```python
from build123d import *

# Parameters (mm, degrees)
F0_W     = 1300
F0_H     = 500
F0_W_2   = 1140
F0_H_2   = 340
F1_DEPTH = 200
F3_DEPTH = 345
F5_DEPTH = 40
F7_DEPTH = 35


# Not quite as in the source:
# - a feature names something its author has since deleted; it is built from what else it names


with BuildPart() as f1:
    # F0 (on Top) → F1 (new body)
    with BuildSketch(Plane.XY):
        Rectangle(F0_W, F0_H)
        Rectangle(F0_W_2, F0_H_2, mode=Mode.SUBTRACT)
    extrude(amount=F1_DEPTH)



with BuildPart() as f3:
    # F2 (on Front) → F3 (new body, symmetric)
    with BuildSketch(Plane.XZ):
        Polygon((1000, 700), (-600, 700), (-1000, 807.1796769724), (-1000, 651.8882499109), (-619.7478746381, 550), (1000, 550), align=None)
    extrude(amount=F3_DEPTH, both=True)


with BuildPart() as f1_1:
    add(f1.part)

    add(f3.part)  # F5 merges F3
    # F4 (on face) → F5 (join)
    with BuildSketch(Plane.XZ.offset(250)):
        Polygon((-385.6647923847, 200), (-450, 170), (-260.7038733478, 170), (-196.3686657325, 200), align=None)
        Polygon((-94.6480633261, 335.7033294112), (-385.6647923847, 200), (-196.3686657325, 200), (0, 291.5682126528), align=None)
        Polygon((-554.2087564458, 550), (-94.6480633261, 335.7033294112), (0, 379.8384461697), (-364.9126297936, 550), align=None)
        Polygon((0, 379.8384461697), (-94.6480633261, 335.7033294112), (0, 291.5682126528), (94.6480633261, 335.7033294112), align=None)
        Polygon((364.9126297936, 550), (0, 379.8384461697), (94.6480633261, 335.7033294112), (554.2087564458, 550), align=None)
        Polygon((94.6480633261, 335.7033294112), (0, 291.5682126528), (196.3686657325, 200), (385.6647923847, 200), align=None)
        Polygon((385.6647923847, 200), (196.3686657325, 200), (260.7038733478, 170), (450, 170), align=None)
    extrude(amount=F5_DEPTH)

    # F6 (on face) → F7 (join)
    with BuildSketch(Plane(origin=(0, 250, 0), x_dir=(-1, 0, 0), z_dir=(0, 1, 0))):
        Polygon((-554.2087564458, 550), (-94.6480633261, 335.7033294113), (0, 379.8384461697), (-364.9126297936, 550), align=None)
        Polygon((364.9126297936, 550), (0, 379.8384461697), (94.6480633261, 335.7033294113), (554.2087564458, 550), align=None)
        Polygon((0, 379.8384461697), (-94.6480633261, 335.7033294113), (0, 291.5682126528), (94.6480633261, 335.7033294113), align=None)
        Polygon((-94.6480633261, 335.7033294113), (-385.6647923847, 200), (-196.3686657325, 200), (0, 291.5682126528), align=None)
        Polygon((94.6480633261, 335.7033294113), (0, 291.5682126528), (196.3686657325, 200), (385.6647923847, 200), align=None)
        Polygon((385.6647923847, 200), (196.3686657325, 200), (260.7038733478, 170), (450, 170), align=None)
        Polygon((-385.6647923847, 200), (-450, 170), (-260.7038733478, 170), (-196.3686657325, 200), align=None)
    extrude(amount=F7_DEPTH)


solid = f1_1.part
```
Geometry check sheet. Reference: the model listing, model coordinates, mm. A direction names the side the tool comes from. Coordinates: 2 decimals unless noted, no trailing zeros. Write each loop counter-clockwise with the first axis right and the second up, starting at its lowest first coordinate (ties: lowest second). Pieces come first, ordered by that corner, then holes. Notation, with made-up numbers: (-7.5, 35) -> (3.5, 35) arc R20 cw to (3.5, 53) -> close; hole circle Ø2 at (57, 4.25). An arc over 180 degrees is marked (long way). Use CSV: the item, a comma, the result in double quotes. Start each with the question number.
Item 1: Depth check by flat-ended pin: pin 1 Ø17.5 at (x, y) = (-383.5, 275.5) entering from -Z; pin 2 Ø12 at (x, y) = (479, -134.5) entering from +Z; pin 3 Ø1 at (x, z) = (49.5, 351) entering from -Y. Enter the tip coordinate at first touch or a pass-through.
Item 2: Set-up check for faces 5 (the flat face through (269.84, 267.26, 254.01)), 6 (the flat face through (321.21, -269.72, 441.35)), 7 (the flat face through (274.811, -269.72, 251.692)), 8 (the flat face through (-8, -170, 99)), 9 (the flat face through (-357, -270, 170)): record each of +Z, -Z, +X, -X, +Y, -Y from which the full face is reachable in a straight line by a thin tool's end or side.
Item 3: Cross-section at A-A, the plane y = -227.5. Record the cut outline in (x, z), plus the area to 3 significant figures.
Item 4: Mould release check, pull along Z, two halves, no side actions. Record for faces 1 (the flat face through (-179.902, -269.72, 463.728)), 2 (the flat face through (650, -3, 99)), 3 (the flat face through (-128.527, 267.255, 231.635)), 4 (the flat face through (179.902, 267.255, 463.728)): released by +Z, released by -Z, zero draft, split by the parting line, or undercut.
Item 5: Cross-section at C-C, the plane z = 149.5. Record the cut outline in (x, y), plus the area to 3 significant figures.
Item 6: Thickness scan on line 1 (Z direction, x = -508, y = 204); line 2 (Y direction, x = 162.5, z = 367.5); line 3 (X direction, y = 143, z = 146.5). Record the ranges inside material, lowest first.
Item 7: Cross-section at D-D, the plane y = 121. Record the cut outline in (x, z).
Item 8: Cross-section at B-B, the plane x = -116.5. Record the cut outline in (y, z).
Answers:
1,pin 1,"z = 170"
1,pin 2,"z = 700"
1,pin 3,"y = -290"
2,face 5,"+X, +Y"
2,face 6,"+X, +Y, -Y"
2,face 7,"+X, -Y"
2,face 8,"-Z"
2,face 9,"-Z, +X, -X, -Y"
3,outline,"(-1000, 651.89) -> (-619.75, 550) -> (1000, 550) -> (1000, 700) -> (-600, 700) -> (-1000, 807.18) -> close; (-650, 0) -> (650, 0) -> (650, 200) -> (-650, 200) -> close"
3,area,"562,000 mm^2"
4,face 1,"undercut"
4,face 2,"zero draft"
4,face 3,"released by -Z"
4,face 4,"undercut"
5,outline,"(-650, -250) -> (650, -250) -> (650, 250) -> (-650, 250) -> close; hole (-570, -170) -> (570, -170) -> (570, 170) -> (-570, 170) -> close"
5,area,"262,000 mm^2"
6,line 1,"0 to 200, 550 to 700"
6,line 2,"-290 to -250, 250 to 285"
6,line 3,"-650 to -570, 570 to 650"
7,outline,"(-1000, 651.89) -> (-619.75, 550) -> (1000, 550) -> (1000, 700) -> (-600, 700) -> (-1000, 807.18) -> close; (-650, 0) -> (-570, 0) -> (-570, 200) -> (-650, 200) -> close; (570, 0) -> (650, 0) -> (650, 200) -> (570, 200) -> close"
8,outline,"(-345, 550) -> (345, 550) -> (345, 700) -> (-345, 700) -> close; (-290, 237.24) -> (-250, 237.24) -> (-250, 325.51) -> (-290, 325.51) -> close; (-290, 345.89) -> (-250, 345.89) -> (-250, 434.16) -> (-290, 434.16) -> close; (-250, 0) -> (-170, 0) -> (-170, 200) -> (-250, 200) -> close; (170, 0) -> (250, 0) -> (250, 200) -> (170, 200) -> close; (250, 237.24) -> (285, 237.24) -> (285, 325.51) -> (250, 325.51) -> close; (250, 345.89) -> (285, 345.89) -> (285, 434.16) -> (250, 434.16) -> close"
